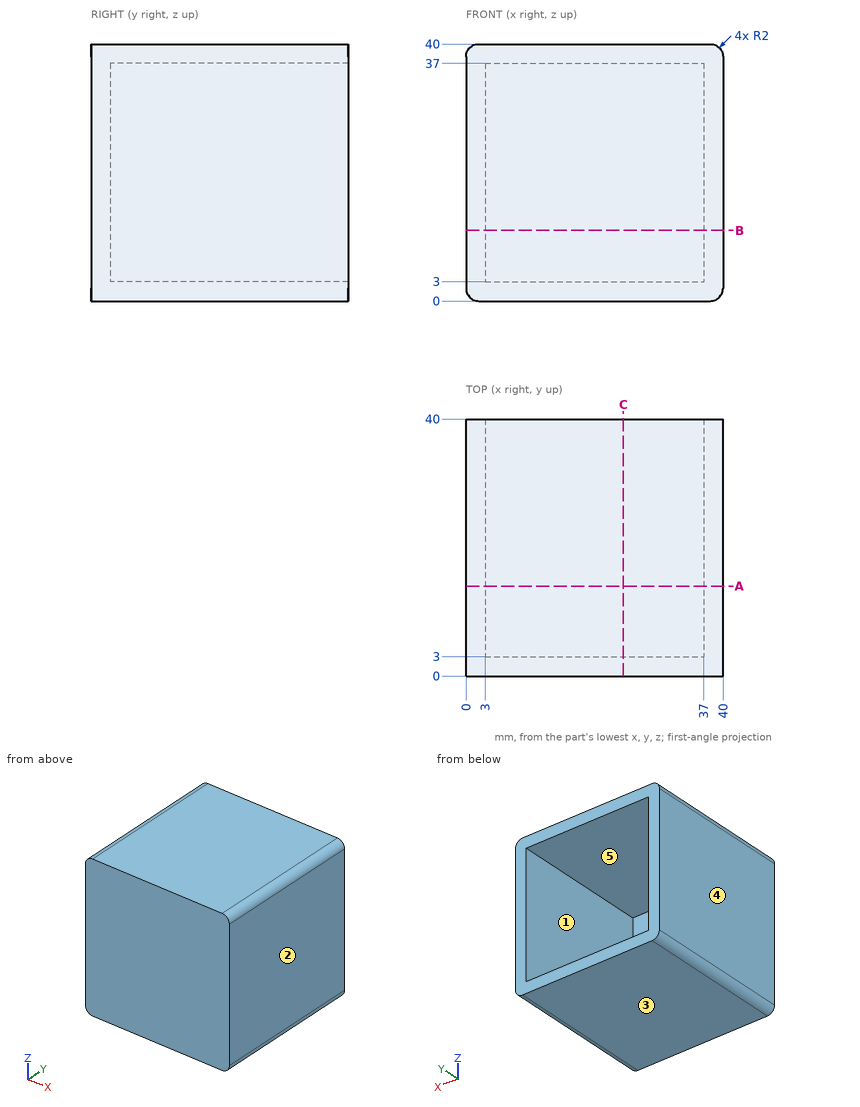
The drawing under review shows one solid part. Ordinate dimensions are in mm from its lowest x, y, z. A direction names the side the tool comes from. Coordinates: 2 decimals unless noted, no trailing zeros. Order: outer loops, then holes, each group sorted by start corner. A loop starts at its lowest first (then second) coordinate and runs counter-clockwise, first axis right, second up. Notation, with made-up numbers: (-15, 30) - (5, 30) arc R17 cw to (5, 60) - close; hole circle Ø8 at (-17.5, -26). An arc over 180 degrees is marked (long way). Put each result on its own line as item: value.
1) The part is to be moulded in two halves that separate along Z. For the marked faces 3, 4 and 5, say which applies: released by +Z, released by -Z, zero draft, split by the parting line, or undercut.
Response values:
face 3: released by -Z
face 4: zero draft
face 5: undercut
2) Wall thickness on L1, parallel to X at y = 33.5, z = 35; L2, parallel to Y at x = 14.5, z = 23: over which ranges is each line inside the solid? List them lowest first. Write a range as from..to.
Response values:
L1: x = 0..3, 37..40
L2: y = 0..3
3) Take a section at A-A, the plane y = 14. Give the boundary of the cut face in (x, z), and give its area (3 significant figures).
Response values:
outline: (0, 2) arc R2 ccw to (2, 0) - (38, 0) arc R2 ccw to (40, 2) - (40, 38) arc R2 ccw to (38, 40) - (2, 40) arc R2 ccw to (0, 38) - close; hole (3, 3) - (37, 3) - (37, 37) - (3, 37) - close
area: 441 mm²
4) Tool access review of the marked faces 1 and 2: name each direction out of +Z, -Z, +X, -X, +Y, -Y from which nothing blocks a thin tool from reaching the whole face with its end or side.
Response values:
face 1: +Y
face 2: +Z, -Z, +X, +Y, -Y
5) Take a section at C-C, the plane x = 24.5. Give the boundary of the cut face in (y, z), and give its area (3 significant figures).
Response values:
outline: (0, 0) - (40, 0) - (40, 3) - (3, 3) - (3, 37) - (40, 37) - (40, 40) - (0, 40) - close
area: 342 mm²
6) Take a section at B-B, the plane z = 11. Give the boundary of the cut face in (x, y).
Response values:
outline: (0, 0) - (40, 0) - (40, 40) - (37, 40) - (37, 3) - (3, 3) - (3, 40) - (0, 40) - close
7) Insertion check: P1, Ø5, axis at x = 18.5, z = 17.5, coming from the +Y side. The pin has a flat end and moves straight along its axis. Give the tip position at first contact, or say it passes through.
Response values:
P1: stops at y = 3
